Can you work these out from the drawing? Everything is in mm from the part's minimum corner. Round coordinates to 2 decimals unless told otherwise and drop trailing zeros. Write each loop counter-clockwise with the first axis right and the second up, starting at its lowest first coordinate (ties: lowest second). Pieces come first, ordered by that corner, then holes. Notation, with made-up numbers: (59, 44.5) -> (68, 44.5) arc R14 ccw to (68, 48.5) -> close; hole circle Ø6 at (61, 72.25). An arc over 180 degrees is marked (long way). One line per question, with ' | ' between items. Start each with the question number.
1. Imagine slicing it at D-D, the plane z = 11. List the corners of the cut face in (x, y) for me.
2. If I drill on line 1 along Z through (x, y) = (9, 1.5); line 2 along X through (y, z) = (1.4, 37.5); line 3 along X through (y, z) = (1.15, 27), over which ranges is the centre line in solid material (lowest first)? Write a range as [from, to].
3. Imagine slicing it at A-A, the plane x = 8. List the corners of the cut face in (y, z) for me.
4. For pin 1 Ø0.6 at (y, z) = (1.5, 20.5) entering from -X; pin 2 Ø2 at (x, z) = (10, 26) entering from -Y; pin 3 Ø0.6 at (y, z) = (1, 27) entering from +X, each with a flat end and sliding along its axis, tell me the tip position at first contact or that it passes through.
5. Imagine slicing it at B-B, the plane z = 37.5. List the corners of the cut face in (x, y) for me.
6. Imagine slicing it at C-C, the plane y = 1.25. List the corners of the cut face in (x, z) for me.
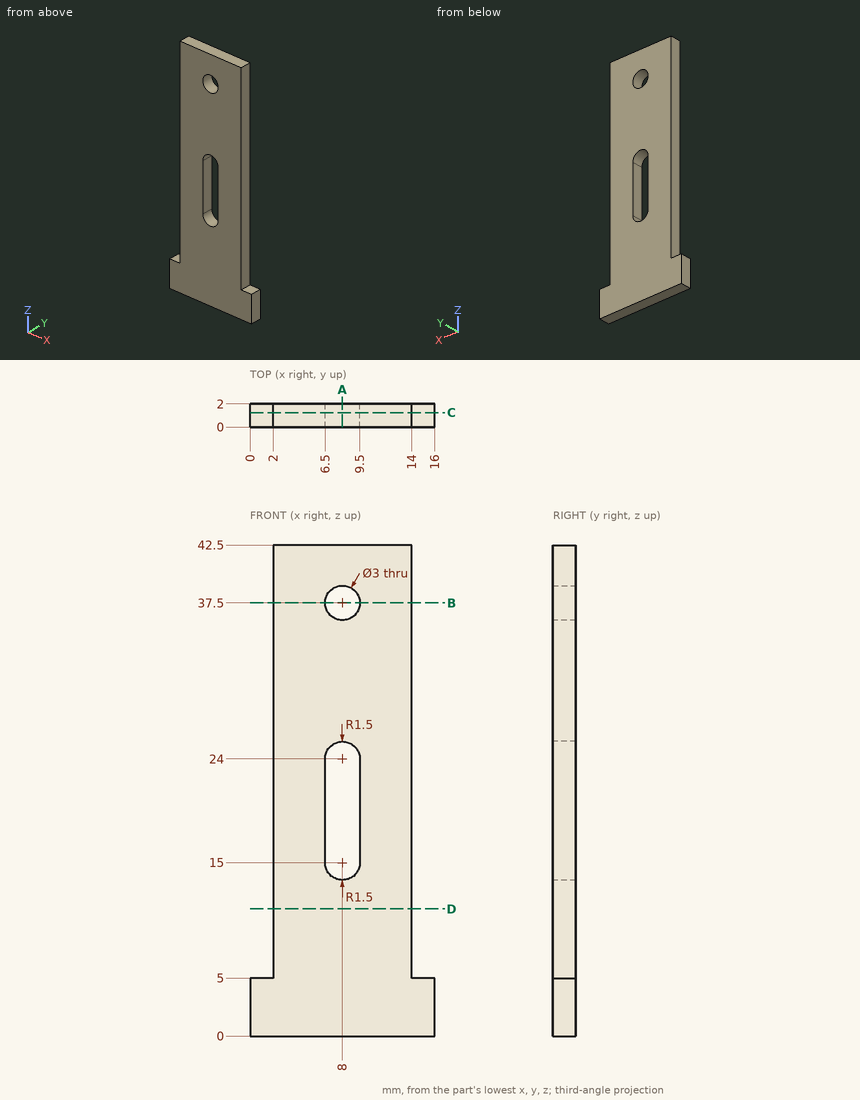
Geometry results:
1) outline: (2, 0) -> (14, 0) -> (14, 2) -> (2, 2) -> close
2) line 1: z = [0, 13.88], [25.12, 36.38], [38.62, 42.5] | line 2: x = [2, 6.5], [9.5, 14] | line 3: x = [2, 14]
3) outline: (0, 0) -> (2, 0) -> (2, 13.5) -> (0, 13.5) -> close; (0, 25.5) -> (2, 25.5) -> (2, 36) -> (0, 36) -> close; (0, 39) -> (2, 39) -> (2, 42.5) -> (0, 42.5) -> close
4) pin 1: stops at x = 2 | pin 2: stops at y = 0 | pin 3: stops at x = 14
5) outline: (2, 0) -> (6.5, 0) -> (6.5, 2) -> (2, 2) -> close; (9.5, 0) -> (14, 0) -> (14, 2) -> (9.5, 2) -> close
6) outline: (0, 0) -> (16, 0) -> (16, 5) -> (14, 5) -> (14, 42.5) -> (2, 42.5) -> (2, 5) -> (0, 5) -> close; hole (6.5, 15) arc R1.5 ccw to (9.5, 15) -> (9.5, 24) arc R1.5 ccw to (6.5, 24) -> close; hole circle Ø3 at (8, 37.5)
